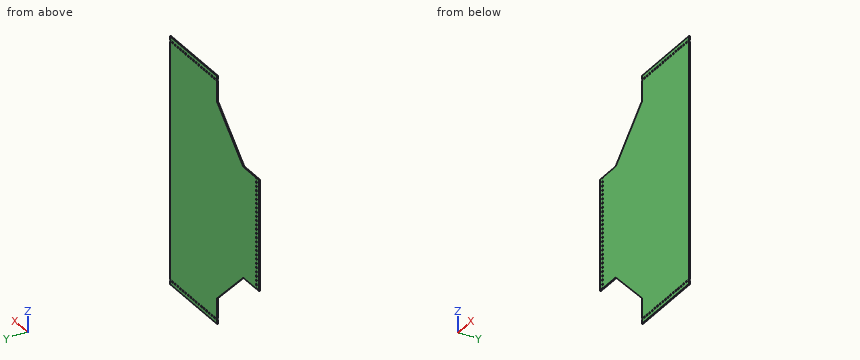
from build123d import *

# Parameters (mm, degrees)
SKETCH1_W                  = 635
SKETCH1_H                  = 736.6
BASE_DEPTH                 = 3.175
SKETCH3_R                  = 2.413
INITIAL_PATTERN_HOLE_DEPTH = 487.272784171
HOLE_PATTERN_1_COUNT       = 58
HOLE_PATTERN_1_PITCH       = 12.7
HOLE_PATTERN_2_OUTLINE_R   = 2.413
HOLE_PATTERN_2_DEPTH       = 3.175
SKETCH4_W                  = 203.2
SKETCH4_H                  = 736.6
TOP_MODULE_CUTOUT_DEPTH    = 487.272784171


# Read off the part's stored shape, not the designer's step: Hole Pattern 2
with BuildPart() as part:
    # Sketch1 → Base (new body)
    with BuildSketch(Plane(origin=(0, 0, 0), x_dir=(1, 0, 0), z_dir=(0, 1, 0))):
        Rectangle(SKETCH1_W, SKETCH1_H)
    extrude(amount=BASE_DEPTH)

    # Sketch3 → Initial Pattern Hole (cut, through all)
    with BuildSketch(Plane(origin=(0, 3.175, 0), x_dir=(1, 0, 0), z_dir=(0, 1, 0))):
        with Locations(Location((-304.8, 355.6, 0), (0, 0, 270))):
            Circle(SKETCH3_R)
        with Locations(Location((304.8, 355.6, 0), (0, 0, 270))):
            Circle(SKETCH3_R)
    initial_pattern_hole = extrude(amount=-INITIAL_PATTERN_HOLE_DEPTH, mode=Mode.SUBTRACT)

    # Hole Pattern 1: Initial Pattern Hole ×58
    with Locations(*[(0, 0, i * HOLE_PATTERN_1_PITCH) for i in range(1, HOLE_PATTERN_1_COUNT)]):
        add(initial_pattern_hole, mode=Mode.SUBTRACT)

    # Hole Pattern 2 outline → Hole Pattern 2 (cut)
    with BuildSketch(Plane(origin=(0, 0, 0), x_dir=(1, 0, 0), z_dir=(0, 1, 0))):
        with Locations((292.1, 355.6)):
            Circle(HOLE_PATTERN_2_OUTLINE_R)
        with Locations((292.1, -355.6)):
            Circle(HOLE_PATTERN_2_OUTLINE_R)
        with Locations((279.4, 355.6)):
            Circle(HOLE_PATTERN_2_OUTLINE_R)
        with Locations((279.4, -355.6)):
            Circle(HOLE_PATTERN_2_OUTLINE_R)
        with Locations((266.7, 355.6)):
            Circle(HOLE_PATTERN_2_OUTLINE_R)
        with Locations((266.7, -355.6)):
            Circle(HOLE_PATTERN_2_OUTLINE_R)
        with Locations((254, 355.6)):
            Circle(HOLE_PATTERN_2_OUTLINE_R)
        with Locations((254, -355.6)):
            Circle(HOLE_PATTERN_2_OUTLINE_R)
        with Locations((241.3, 355.6)):
            Circle(HOLE_PATTERN_2_OUTLINE_R)
        with Locations((241.3, -355.6)):
            Circle(HOLE_PATTERN_2_OUTLINE_R)
        with Locations((228.6, 355.6)):
            Circle(HOLE_PATTERN_2_OUTLINE_R)
        with Locations((228.6, -355.6)):
            Circle(HOLE_PATTERN_2_OUTLINE_R)
        with Locations((215.9, 355.6)):
            Circle(HOLE_PATTERN_2_OUTLINE_R)
        with Locations((215.9, -355.6)):
            Circle(HOLE_PATTERN_2_OUTLINE_R)
        with Locations((203.2, 355.6)):
            Circle(HOLE_PATTERN_2_OUTLINE_R)
        with Locations((203.2, -355.6)):
            Circle(HOLE_PATTERN_2_OUTLINE_R)
        with Locations((190.5, 355.6)):
            Circle(HOLE_PATTERN_2_OUTLINE_R)
        with Locations((190.5, -355.6)):
            Circle(HOLE_PATTERN_2_OUTLINE_R)
        with Locations((177.8, 355.6)):
            Circle(HOLE_PATTERN_2_OUTLINE_R)
        with Locations((177.8, -355.6)):
            Circle(HOLE_PATTERN_2_OUTLINE_R)
        with Locations((165.1, 355.6)):
            Circle(HOLE_PATTERN_2_OUTLINE_R)
        with Locations((165.1, -355.6)):
            Circle(HOLE_PATTERN_2_OUTLINE_R)
        with Locations((152.4, 355.6)):
            Circle(HOLE_PATTERN_2_OUTLINE_R)
        with Locations((152.4, -355.6)):
            Circle(HOLE_PATTERN_2_OUTLINE_R)
        with Locations((139.7, 355.6)):
            Circle(HOLE_PATTERN_2_OUTLINE_R)
        with Locations((139.7, -355.6)):
            Circle(HOLE_PATTERN_2_OUTLINE_R)
        with Locations((127, 355.6)):
            Circle(HOLE_PATTERN_2_OUTLINE_R)
        with Locations((127, -355.6)):
            Circle(HOLE_PATTERN_2_OUTLINE_R)
        with Locations((114.3, 355.6)):
            Circle(HOLE_PATTERN_2_OUTLINE_R)
        with Locations((114.3, -355.6)):
            Circle(HOLE_PATTERN_2_OUTLINE_R)
        with Locations((101.6, 355.6)):
            Circle(HOLE_PATTERN_2_OUTLINE_R)
        with Locations((101.6, -355.6)):
            Circle(HOLE_PATTERN_2_OUTLINE_R)
        with Locations((88.9, 355.6)):
            Circle(HOLE_PATTERN_2_OUTLINE_R)
        with Locations((88.9, -355.6)):
            Circle(HOLE_PATTERN_2_OUTLINE_R)
        with Locations((76.2, 355.6)):
            Circle(HOLE_PATTERN_2_OUTLINE_R)
        with Locations((76.2, -355.6)):
            Circle(HOLE_PATTERN_2_OUTLINE_R)
        with Locations((63.5, 355.6)):
            Circle(HOLE_PATTERN_2_OUTLINE_R)
        with Locations((63.5, -355.6)):
            Circle(HOLE_PATTERN_2_OUTLINE_R)
        with Locations((50.8, 355.6)):
            Circle(HOLE_PATTERN_2_OUTLINE_R)
        with Locations((50.8, -355.6)):
            Circle(HOLE_PATTERN_2_OUTLINE_R)
        with Locations((38.1, 355.6)):
            Circle(HOLE_PATTERN_2_OUTLINE_R)
        with Locations((38.1, -355.6)):
            Circle(HOLE_PATTERN_2_OUTLINE_R)
        with Locations((25.4, 355.6)):
            Circle(HOLE_PATTERN_2_OUTLINE_R)
        with Locations((25.4, -355.6)):
            Circle(HOLE_PATTERN_2_OUTLINE_R)
        with Locations((12.7, 355.6)):
            Circle(HOLE_PATTERN_2_OUTLINE_R)
        with Locations((12.7, -355.6)):
            Circle(HOLE_PATTERN_2_OUTLINE_R)
        with Locations((0, 355.6)):
            Circle(HOLE_PATTERN_2_OUTLINE_R)
        with Locations((0, -355.6)):
            Circle(HOLE_PATTERN_2_OUTLINE_R)
        with Locations((-12.7, 355.6)):
            Circle(HOLE_PATTERN_2_OUTLINE_R)
        with Locations((-12.7, -355.6)):
            Circle(HOLE_PATTERN_2_OUTLINE_R)
        with Locations((-25.4, 355.6)):
            Circle(HOLE_PATTERN_2_OUTLINE_R)
        with Locations((-25.4, -355.6)):
            Circle(HOLE_PATTERN_2_OUTLINE_R)
        with Locations((-38.1, 355.6)):
            Circle(HOLE_PATTERN_2_OUTLINE_R)
        with Locations((-38.1, -355.6)):
            Circle(HOLE_PATTERN_2_OUTLINE_R)
        with Locations((-50.8, 355.6)):
            Circle(HOLE_PATTERN_2_OUTLINE_R)
        with Locations((-50.8, -355.6)):
            Circle(HOLE_PATTERN_2_OUTLINE_R)
        with Locations((-63.5, 355.6)):
            Circle(HOLE_PATTERN_2_OUTLINE_R)
        with Locations((-63.5, -355.6)):
            Circle(HOLE_PATTERN_2_OUTLINE_R)
        with Locations((-76.2, 355.6)):
            Circle(HOLE_PATTERN_2_OUTLINE_R)
        with Locations((-76.2, -355.6)):
            Circle(HOLE_PATTERN_2_OUTLINE_R)
        with Locations((-88.9, 355.6)):
            Circle(HOLE_PATTERN_2_OUTLINE_R)
        with Locations((-88.9, -355.6)):
            Circle(HOLE_PATTERN_2_OUTLINE_R)
        with Locations((-101.6, 355.6)):
            Circle(HOLE_PATTERN_2_OUTLINE_R)
        with Locations((-101.6, -355.6)):
            Circle(HOLE_PATTERN_2_OUTLINE_R)
        with Locations((-114.3, 355.6)):
            Circle(HOLE_PATTERN_2_OUTLINE_R)
        with Locations((-114.3, -355.6)):
            Circle(HOLE_PATTERN_2_OUTLINE_R)
        with Locations((-127, 355.6)):
            Circle(HOLE_PATTERN_2_OUTLINE_R)
        with Locations((-127, -355.6)):
            Circle(HOLE_PATTERN_2_OUTLINE_R)
        with Locations((-139.7, 355.6)):
            Circle(HOLE_PATTERN_2_OUTLINE_R)
        with Locations((-139.7, -355.6)):
            Circle(HOLE_PATTERN_2_OUTLINE_R)
        with Locations((-152.4, 355.6)):
            Circle(HOLE_PATTERN_2_OUTLINE_R)
        with Locations((-152.4, -355.6)):
            Circle(HOLE_PATTERN_2_OUTLINE_R)
        with Locations((-165.1, 355.6)):
            Circle(HOLE_PATTERN_2_OUTLINE_R)
        with Locations((-165.1, -355.6)):
            Circle(HOLE_PATTERN_2_OUTLINE_R)
        with Locations((-177.8, 355.6)):
            Circle(HOLE_PATTERN_2_OUTLINE_R)
        with Locations((-177.8, -355.6)):
            Circle(HOLE_PATTERN_2_OUTLINE_R)
        with Locations((-190.5, 355.6)):
            Circle(HOLE_PATTERN_2_OUTLINE_R)
        with Locations((-190.5, -355.6)):
            Circle(HOLE_PATTERN_2_OUTLINE_R)
        with Locations((-203.2, 355.6)):
            Circle(HOLE_PATTERN_2_OUTLINE_R)
        with Locations((-203.2, -355.6)):
            Circle(HOLE_PATTERN_2_OUTLINE_R)
        with Locations((-215.9, 355.6)):
            Circle(HOLE_PATTERN_2_OUTLINE_R)
        with Locations((-215.9, -355.6)):
            Circle(HOLE_PATTERN_2_OUTLINE_R)
        with Locations((-228.6, 355.6)):
            Circle(HOLE_PATTERN_2_OUTLINE_R)
        with Locations((-228.6, -355.6)):
            Circle(HOLE_PATTERN_2_OUTLINE_R)
        with Locations((-241.3, 355.6)):
            Circle(HOLE_PATTERN_2_OUTLINE_R)
        with Locations((-241.3, -355.6)):
            Circle(HOLE_PATTERN_2_OUTLINE_R)
        with Locations((-254, 355.6)):
            Circle(HOLE_PATTERN_2_OUTLINE_R)
        with Locations((-254, -355.6)):
            Circle(HOLE_PATTERN_2_OUTLINE_R)
        with Locations((-266.7, 355.6)):
            Circle(HOLE_PATTERN_2_OUTLINE_R)
        with Locations((-266.7, -355.6)):
            Circle(HOLE_PATTERN_2_OUTLINE_R)
        with Locations((-279.4, 355.6)):
            Circle(HOLE_PATTERN_2_OUTLINE_R)
        with Locations((-279.4, -355.6)):
            Circle(HOLE_PATTERN_2_OUTLINE_R)
        with Locations((-292.1, 355.6)):
            Circle(HOLE_PATTERN_2_OUTLINE_R)
        with Locations((-292.1, -355.6)):
            Circle(HOLE_PATTERN_2_OUTLINE_R)
    extrude(amount=HOLE_PATTERN_2_DEPTH, mode=Mode.SUBTRACT)

    # Sketch4 → Top Module Cutout (cut, through all)
    with BuildSketch(Plane(origin=(0, 3.175, 0), x_dir=(1, 0, 0), z_dir=(0, 1, 0))):
        Polygon((-317.5, 165.1), (-241.3, 165.1), (-114.3, 292.1), (-114.3, 368.3), (-317.5, 368.3), align=None)
        Polygon((-317.5, -368.3), (-114.3, -368.3), (-114.3, -292.1), (-241.3, -165.1), (-317.5, -165.1), align=None)
        with Locations((215.9, 0)):
            Rectangle(SKETCH4_W, SKETCH4_H)
    extrude(amount=-TOP_MODULE_CUTOUT_DEPTH, mode=Mode.SUBTRACT)


solid = part.part
Work out the finished part from the listing and answer in its coordinate system (mm). Coordinates: 2 decimals unless noted, no trailing zeros. Write each loop counter-clockwise with the first axis right and the second up, starting at its lowest first coordinate (ties: lowest second). Pieces come first, ordered by that corner, then holes. Notation, with made-up numbers: M -39,26.5 L -10,26.5 A27 cw -10,51.5 Z; hole C -6.75,45.25 d10. An arc over 180 degrees is marked long. Use one line per item in the form item = value. Start each with the question number.
1. Straight lines are drawn through the part: probe 1 along X at (y, z) = (0.35, 75.5); probe 2 along Z at (x, y) = (91, 0.5); probe 3 along X at (y, z) = (2.1, 102). For each, find the intervals that lie inside material, in ascending order. Write a range as from..to.
2. The part is cut by section C-C (y = 1.5). Give the number of separate pieces and of enclosed holes in the cut face, plus the area to 3 significant figures.
3. Each of these flat-tipped pins is pushed along its axis until it touches: P1, Ø1.5, axis at x = -271.5, y = 0.5, coming from the -Z side; P2, Ø1.6, axis at y = 2, z = 310, coming from the -X side; P3, Ø1, axis at x = -148.5, y = 1.5, coming from the -Z side. Where does it stop, or does it pass through?
4. The part is cut by section B-B (x = -180). Give the vertices of the cut face in (y, z) (3 decimals), plus the area to 3 significant figures.
5. The part is cut by section A-A (z = 185). Give the vertices of the cut face in (x, y) (3 decimals).
Evaluation:
q1.probe_1 = -317.5..-307.11, -302.49..114.3
q1.probe_2 = -368.3..-356.79, -354.41..354.41, 356.79..368.3
q1.probe_3 = -317.5..-307.18, -302.42..114.3
q2.separate_pieces = 1
q2.enclosed_holes = 59
q2.area = 250,000 mm^2
q3.P1 = -165.1
q3.P2 = -114.3
q3.P3 = -258.4
q4.outline = M 0,-226.4 L 3.175,-226.4 L 3.175,226.4 L 0,226.4 Z
q4.area = 1,440 mm^2
q5.outline = M -221.4,0 L 114.3,0 L 114.3,3.175 L -221.4,3.175 Z
